Autodesk Inventor part; units mm, degrees
ref_plane "YZ Plane" through (0, 0, 0) normal (1, 0, 0) x (0, 1, 0)
ref_plane "XZ Plane" through (0, 0, 0) normal (0, 1, 0) x (-1, 0, 0)
ref_plane "XY Plane" through (0, 0, 0) normal (0, 0, 1) x (1, 0, 0)
sketch "Boceto2" plane through (0, 0, 0) normal (0, 0, 1) x (1, 0, 0)
  circle A0 centre (0, 0) radius 40
  circle A1 centre (-200, 0) radius 52.5
  circle A2 centre (-250, -5) radius 40
  arc A3 (-258.4353, -44.1005) -> (-204.7198, -52.2874) centre (-164.804, 389.9147) ccw
  arc A4 (-188.9974, 51.3341) -> (-279.8859, 21.5863) centre (-208.9069, -41.5562) ccw
  arc A5 (-179.4312, 48.3029) -> (-11.2392, 38.3885) centre (-81.4844, 278.3169) ccw
  arc A6 (-46.5935, -31) -> (31.225, 25) centre (-6.245, -5) ccw
  arc A7 (-18.0162, -51.5343) -> (-187.4585, -50.98) centre (-103.8482, -390.8466) ccw
  dimension "d42" = 80
  dimension "d43" = 200
  dimension "d44" = 105
  dimension "d45" = 80
  dimension "d46" = 50
  dimension "d47" = 5
  dimension "d48" = 444
  dimension "d49" = 95
  dimension "d50" = 250
  dimension "d51" = 350
  dimension "d52" = 5
  dimension "d53" = 48
  dimension "d54" = 31
extrude "Extrusión1" add sketch "Boceto2" along normal blind 3.3
sketch "Boceto3" plane through (0, 0, 3.3) normal (0, 0, 1) x (1, 0, 0)
  arc A0 (-179.4312, 48.3029) -> (-11.2392, 38.3885) centre (-81.4844, 278.3169) ccw
  arc A1 (31.225, 25) -> (-11.2392, 38.3885) centre (0, 0) ccw
  arc A2 (-179.4312, 48.3029) -> (-11.2392, 38.3885) centre (-81.4844, 278.3169) ccw
  arc A3 (-179.4312, 48.3029) -> (-188.9974, 51.3341) centre (-200, 0) ccw
  arc A4 (-188.9974, 51.3341) -> (-279.8859, 21.5863) centre (-208.9069, -41.5562) ccw
  arc A5 (-279.8859, 21.5863) -> (-258.4353, -44.1005) centre (-250, -5) ccw
  arc A6 (-258.4353, -44.1005) -> (-204.7198, -52.2874) centre (-164.804, 389.9147) ccw
  arc A7 (-204.7198, -52.2874) -> (-187.4585, -50.98) centre (-200, 0) ccw
  arc A8 (-18.0162, -51.5343) -> (-187.4585, -50.98) centre (-103.8482, -390.8466) ccw
  arc A9 (-18.0162, -51.5343) -> (31.225, 25) centre (-6.245, -5) ccw
  arc A10 (-18.0162, -51.5343) -> (31.225, 25) centre (-6.245, -5) ccw
  arc A11 (31.225, 25) -> (-11.2392, 38.3885) centre (0, 0) ccw
  line L0 (1.755, 39.9615) -> (41.755, -5.0385)
  arc A12 (-279.8859, 21.5863) -> (-258.4353, -44.1005) centre (-250, -5) ccw
  line L1 (-288.1379, 7.0623) -> (-243.1379, 47.0623)
  arc A13 (-188.9974, 51.3341) -> (-279.8859, 21.5863) centre (-208.9069, -41.5562) ccw
  line L2 (-7.2418, 4.9269) -> (19.3327, -24.9694)
  line L3 (19.3327, -24.9694) -> (4.3845, -38.2567)
  line L4 (4.3845, -38.2567) -> (-22.19, -8.3603)
  line L5 (-22.19, -8.3603) -> (-7.2418, 4.9269)
  line L6 (-268.207, -15.36) -> (-254.9197, -30.3082)
  line L7 (-254.9197, -30.3082) -> (-225.0234, -3.7336)
  line L8 (-225.0234, -3.7336) -> (-238.3106, 11.2146)
  line L9 (-268.207, -15.36) -> (-238.3106, 11.2146)
  line L10 (-265.7987, -10.5434) -> (-220.9541, 29.3185)
  line L11 (-223.1465, 31.7849) -> (-267.9911, -8.0769)
  line L12 (-249.854, -28.4812) -> (-205.0094, 11.3807)
  line L13 (-205.0094, 11.3807) -> (-202.817, 8.9142)
  line L14 (-202.817, 8.9142) -> (-247.6616, -30.9476)
  line L15 (-247.6616, -30.9476) -> (-249.854, -28.4812)
  circle A14 centre (-228.1168, 6.8962) radius 1
  circle A15 centre (-265.1136, -25.9898) radius 1
  line L16 (-22.3561, 24.9409) -> (17.5057, -19.9037)
  line L17 (17.5057, -19.9037) -> (19.9722, -17.7113)
  line L18 (19.9722, -17.7113) -> (-19.8897, 27.1333)
  line L19 (-19.8897, 27.1333) -> (-22.3561, 24.9409)
  line L20 (-40.2939, 8.9962) -> (-0.4321, -35.8484)
  line L21 (-0.4321, -35.8484) -> (-2.8986, -38.0408)
  line L22 (-2.8986, -38.0408) -> (-42.7604, 6.8038)
  line L23 (-42.7604, 6.8038) -> (-40.2939, 8.9962)
  circle A16 centre (-17.8717, 1.8335) radius 1
  circle A17 centre (15.0143, -35.1633) radius 1
  arc A18 (-18.0162, -51.5343) -> (-187.4585, -50.98) centre (-103.8482, -390.8466) ccw
  line L24 (-220.9541, 29.3185) -> (-223.1465, 31.7849)
  line L25 (-267.9911, -8.0769) -> (-265.7987, -10.5434)
  line L26 (-253.2588, -2.0727) -> (-239.9715, -17.0209) construction
  line L27 (-8.9028, -23.3085) -> (6.0454, -10.0212) construction
  line L28 (-225, -34) -> (-25, -34)
  line L29 (-25, -34) -> (-25, -37)
  line L30 (-25, -37) -> (-225, -37)
  line L31 (-225, -37) -> (-225, -34)
  dimension "d59" = 40
  dimension "d60" = 45
  dimension "d61" = 40
  dimension "d62" = 45
  dimension "d65" = 40
  dimension "d66" = 20
  dimension "d68" = 30
  dimension "d69" = 0
  dimension "d70" = 40
  dimension "d71" = 20
  dimension "d73" = 30
  dimension "d74" = 0
  dimension "d75" = 2
  dimension "d76" = 2
  dimension "d77" = 3.3
  dimension "d78" = 3.3
  dimension "d80" = 60
  dimension "d84" = 2
  dimension "d85" = 2
  dimension "d86" = 4.75
  dimension "d87" = 10
  dimension "d88" = 4.75
  dimension "d89" = 10
  dimension "d90" = 2
  dimension "d91" = 2
  dimension "d94" = 3.3
  dimension "d95" = 3.3
  dimension "d96" = 60
  dimension "d97" = 60
  dimension "d98" = 2
  dimension "d99" = 10
  dimension "d100" = 10
  dimension "d101" = 4.75
  dimension "d102" = 4.75
  dimension "d103" = 60
  dimension "d105" = 15
  dimension "d106" = 15
  dimension "d107" = 15
  dimension "d108" = 15
  dimension "d109" = 3
  dimension "d110" = 34
  dimension "d111" = 200
  dimension "d112" = 25
extrude "Extrusión2" cut sketch "Boceto3" against normal blind 3.3 contours A1 A9 L0 | L1 A5 A4 | L2 L3 L4 L5 | L9 L8 L7 L6 | L25 L11 L24 L10 | L12 L13 L14 L15 | A14 | A15 | L19 L18 L17 L16 | L20 L21 L22 L23 | A16 | A17 | L28 L29 L30 L31
sketch "Sketch4" plane through (0, 0, 3.3) normal (0, 0, 1) x (1, 0, 0)
  arc A0 (-179.4312, 48.3029) -> (-11.2392, 38.3885) centre (-81.4844, 278.3169) ccw
  line L0 (-225, -34) -> (-25, -34)
  arc A1 (-179.4312, 48.3029) -> (-188.9974, 51.3341) centre (-200, 0) ccw
  arc A2 (-188.9974, 51.3341) -> (-243.1379, 47.0623) centre (-208.9069, -41.5562) ccw
  line L1 (-209.9139, -26) -> (-238.1379, -26)
  line L2 (41.755, -5.0385) -> (1.755, 39.9615)
  arc A3 (1.755, 39.9615) -> (-11.2392, 38.3885) centre (0, 0) ccw
  arc A4 (-179.4312, 48.3029) -> (-11.2392, 38.3885) centre (-81.4844, 278.3169) ccw
  arc A5 (-179.4312, 48.3029) -> (-188.9974, 51.3341) centre (-200, 0) ccw
  arc A6 (-188.9974, 51.3341) -> (-243.1379, 47.0623) centre (-208.9069, -41.5562) ccw
  line L3 (-243.1379, 47.0623) -> (-288.1379, 7.0623)
  arc A7 (-288.1379, 7.0623) -> (-258.4353, -44.1005) centre (-250, -5) ccw
  arc A8 (-258.4353, -44.1005) -> (-204.7198, -52.2874) centre (-164.804, 389.9147) ccw
  arc A9 (-204.7198, -52.2874) -> (-187.4585, -50.98) centre (-200, 0) ccw
  arc A10 (-18.0162, -51.5343) -> (-187.4585, -50.98) centre (-103.8482, -390.8466) ccw
  arc A11 (-18.0162, -51.5343) -> (41.755, -5.0385) centre (-6.245, -5) ccw
  line L4 (-225.0234, -3.7336) -> (-254.9197, -30.3082)
  line L5 (-254.9197, -30.3082) -> (-268.207, -15.36)
  line L6 (-268.207, -15.36) -> (-238.3106, 11.2146)
  line L7 (-238.3106, 11.2146) -> (-225.0234, -3.7336)
  line L8 (-247.6616, -30.9476) -> (-249.854, -28.4812)
  line L9 (-249.854, -28.4812) -> (-205.0094, 11.3807)
  line L10 (-205.0094, 11.3807) -> (-202.817, 8.9142)
  line L11 (-202.817, 8.9142) -> (-247.6616, -30.9476)
  line L12 (19.9722, -17.7113) -> (17.5057, -19.9037)
  line L13 (17.5057, -19.9037) -> (-22.3561, 24.9409)
  line L14 (-22.3561, 24.9409) -> (-19.8897, 27.1333)
  line L15 (-19.8897, 27.1333) -> (19.9722, -17.7113)
  circle A12 centre (15.0143, -35.1633) radius 1
  circle A13 centre (-265.1136, -25.9898) radius 1
  circle A14 centre (-228.1168, 6.8962) radius 1
  circle A15 centre (-17.8717, 1.8335) radius 1
  line L16 (-42.7604, 6.8038) -> (-40.2939, 8.9962)
  line L17 (-40.2939, 8.9962) -> (-0.4321, -35.8484)
  line L18 (-0.4321, -35.8484) -> (-2.8986, -38.0408)
  line L19 (-2.8986, -38.0408) -> (-42.7604, 6.8038)
  line L20 (-223.1465, 31.7849) -> (-220.9541, 29.3185)
  line L21 (-220.9541, 29.3185) -> (-265.7987, -10.5434)
  line L22 (-265.7987, -10.5434) -> (-267.9911, -8.0769)
  line L23 (-267.9911, -8.0769) -> (-223.1465, 31.7849)
  line L24 (-22.19, -8.3603) -> (-7.2418, 4.9269)
  line L25 (-7.2418, 4.9269) -> (19.3327, -24.9694)
  line L26 (19.3327, -24.9694) -> (4.3845, -38.2567)
  line L27 (4.3845, -38.2567) -> (-22.19, -8.3603)
  line L28 (-225, -37) -> (-225, -34)
  line L29 (-225, -34) -> (-25, -34)
  line L30 (-25, -34) -> (-25, -37)
  line L31 (-25, -37) -> (-225, -37)
  line L32 (-202.817, 8.9142) -> (-247.6616, -30.9476)
  arc A16 (-238.3772, -25.3707) -> (-238.1379, -26) centre (-238.1379, -25.6399) ccw
  line L33 (-238.3772, -25.3707) -> (-222.7894, -11.515)
  line L34 (-222.7894, -11.515) -> (-209.9139, -26)
  line L35 (-196.5343, -26) -> (-215.3153, -4.8713)
  line L36 (-215.3153, -4.8713) -> (-207.8412, 1.7723)
  line L37 (-207.8412, 1.7723) -> (-183.1548, -26)
  line L38 (-183.1548, -26) -> (-196.5343, -26)
  line L39 (-200.3672, 8.4159) -> (-169.7752, -26)
  line L40 (-200.3672, 8.4159) -> (-179.974, 26.5432)
  arc A17 (-160.6008, 30.6466) -> (-179.974, 26.5432) centre (-166.6867, 11.595) ccw
  arc A18 (-160.6008, 30.6466) -> (-56.7209, 19.4989) centre (-81.4844, 278.3169) ccw
  line L41 (-56.7209, 19.4989) -> (-45.4609, 6.8314)
  arc A19 (-103.245, -26) -> (-38.6081, -0.8779) centre (-182.2347, 272.9473) ccw
  line L42 (-267.9911, -8.0769) -> (-223.1465, 31.7849)
  arc A20 (-18.0162, -51.5343) -> (41.755, -5.0385) centre (-6.245, -5) ccw
  line L43 (-103.245, -26) -> (-33.245, -26)
  arc A21 (-33.245, -26) -> (-27.5501, -13.3183) centre (-33.245, -18.3804) ccw
  line L44 (-38.6081, -0.8779) -> (-27.5501, -13.3183)
  line L45 (-2.8986, -38.0408) -> (-42.7604, 6.8038)
  line L46 (-42.7604, 6.8038) -> (-40.2939, 8.9962)
  arc A22 (-169.7752, -26) -> (-45.4609, 6.8314) centre (-182.2347, 272.9473) ccw
  line L47 (-223.1465, 31.7849) -> (-220.9541, 29.3185)
  dimension "d113" = 10
  dimension "d114" = 10
  dimension "d115" = 10
  dimension "d117" = 10
  dimension "d119" = 50
  dimension "d121" = 10
  dimension "d126" = 10
  dimension "d129" = 10
  dimension "d130" = 75
  dimension "d131" = 70
  dimension "d132" = 20
  dimension "d136" = 10
  dimension "d139" = 10
extrude "Extrusión5" cut sketch "Sketch4" against normal blind 10 contours L1 A16 L33 L34 | L35 L36 L37 L38 | L40 A17 A18 L41 A22 L39 | A19 L44 A21 L43
equation "\"d45\" = d42"
equation "\"d65\" = altura_servo"
equation "\"d66\" = base_servo"
equation "\"d70\" = d65"
equation "\"d71\" = d66"
equation "\"d78\" = d77"
equation "\"d84\" = agujero_servo"
equation "\"d85\" = d84"
equation "\"d87\" = 0.5 * d71"
equation "\"d88\" = d86"
equation "\"d89\" = 0.5 * d71"
equation "\"d91\" = d90"
equation "\"d95\" = d94"
equation "\"d97\" = d96"
equation "\"d98\" = agujero_servo"
equation "\"d99\" = 0.5 * d66"
equation "\"d100\" = d99"
equation "\"d102\" = d101"
equation "\"soporte\" = 60"
equation "\"largo_base\" = 200"
properties part number "Cuerpo - Lateral"
CAD build for the part. Positions are in the model's coordinates, mm. A direction names the side the tool comes from. Round coordinates to 2 decimals unless told otherwise and drop trailing zeros. Order: outer loops, then holes, each group sorted by start corner. A loop starts at its lowest first (then second) coordinate and runs counter-clockwise, first axis right, second up.
Item 1: Tool access for faces 4 (the face through (-26.345, -21.613, 1.673)), 5 (the face through (-216.76, 53.12, 1.63)): list every direction of +Z, -Z, +X, -X, +Y, -Y with a clear straight run to the whole face (end or side of a thin tool).
Item 2: Probe line 1 along X through (y, z) = (-31, 3.1); line 2 along Y through (x, z) = (-226, 2.75); line 3 along X through (y, z) = (-31.5, 3.15). List the from-to ranges inside material, lowest first.
Item 3: Pin check, flat tips, straight feed: pin 1 (1.6 mm diameter, centred on x = -227.5, z = 2, fed in from +Y); pin 2 (1 mm diameter, centred on x = 7.5, z = 2.5, fed in from -Y); pin 3 (1.6 mm diameter, centred on x = -110, z = 2.5, fed in from +Y). Stop position of each tip, or through.
Item 4: Saw through at A-A on x = -176.5. Write the cut outline in (y, z).
Item 5: Saw through at C-C on z = 1.3. State how many separate pieces and enclosed holes the cut face has, then the cut area to 3 significant figures.
Item 6: Saw through at D-D on y = 44. Write the cut outline in (x, z), then the cut area to 3 significant figures.
Item 7: Saw through at B-B on x = -74. Write the cut outline in (y, z), then the cut area to 3 significant figures.
Item 8: Mould opens along X. For faces 1 (the face through (-261.656, -22.729, 1.673)), 2 (the face through (-126, 25, 3.3)), 3 (the face through (21.47, 17.78, 1.67)) say: pulls with the +X half, pulls with the -X half, needs draft (parallel to the pull), parting line crosses it, or undercut.
Reported:
1. face 4: +Z, -Z
1. face 5: +Z, -Z, +Y
2. line 1: x = -280.4 to -9.16, -4.74 to -2.07, 12.55 to 34.1
2. line 2: y = -49.85 to -26, -14.37 to -11.69, -7.28 to -4.6, -2.63 to 24.83, 29.25 to 51.89
2. line 3: x = -279.96 to -8.71, -4.3 to -1.62, 11.99 to 33.78
3. pin 1: stops at y = 51.76
3. pin 2: stops at y = -51.14
3. pin 3: stops at y = 30.04
4. outline: (-48.47, 0) - (-37, 0) - (-37, 3.3) - (-48.47, 3.3) - close; (-34, 0) - (-18.43, 0) - (-18.43, 3.3) - (-34, 3.3) - close; (29.02, 0) - (47.08, 0) - (47.08, 3.3) - (29.02, 3.3) - close
5. separate pieces: 1
5. enclosed holes: 15
5. area: 16,300 mm2
6. outline: (-246.58, 0) - (-168.64, 0) - (-168.64, 3.3) - (-246.58, 3.3) - close
6. area: 257 mm2
7. outline: (-42.12, 0) - (-37, 0) - (-37, 3.3) - (-42.12, 3.3) - close; (-34, 0) - (-26, 0) - (-26, 3.3) - (-34, 3.3) - close; (-16.7, 0) - (-6, 0) - (-6, 3.3) - (-16.7, 3.3) - close; (18.42, 0) - (28.43, 0) - (28.43, 3.3) - (18.42, 3.3) - close
7. area: 112 mm2
8. face 1: undercut
8. face 2: needs draft
8. face 3: pulls with the +X half
